For this review, take the finished solid that the model builds, in its own axes (mm). Face numbers are marked on the shaded views. A direction names the side the tool comes from. Give positions to 0.01 mm unless a question says otherwise; leave off trailing zeros. Loops run counter-clockwise (first coordinate to the right, second up) from the corner with the lowest first, then second, coordinate; pieces in that order, holes last. Notation, with made-up numbers: M 67.25,59 L 107.25,59 A16 ccw 107.25,65 Z; hole C -12.75,49 d5. An arc over 180 degrees is marked long. Use CSV: the item, a comma, the result in double quotes. Start each with the question number.
1. Insertion check: P1, Ø2, axis at x = 48.5, y = 26.5, coming from the +Z side; P2, Ø1.5, axis at y = 4.5, z = -7, coming from the -X side (3 decimals); P3, Ø6, axis at y = 18.5, z = -7, coming from the +X side (3 decimals). Each pin has a flat end and moves straight along its axis. Give the tip position at first contact, or say it passes through.
2. Take a section at C-C, the plane y = 7.5. Write out the cut boundary in (x, z) (3 decimals).
3. The part is to be moulded in two halves that separate along Y. For the marked faces 1, 2 and 3, say which applies: pulls with the +Y half, pulls with the -Y half, needs draft (parallel to the pull), parting line crosses it, or undercut.
4. Take a section at D-D, the plane y = -54.5. Write out the cut boundary in (x, z).
5. Take a section at B-B, the plane x = 39. Write out the cut boundary in (y, z), and give its area (3 significant figures).
6. Tool access review of the marked faces 4, 5 and 6: name each direction out of +Z, -Z, +X, -X, +Y, -Y from which nothing blocks a thin tool from reaching the whole face with its end or side.
7. Take a section at A-A, the plane z = -13. Write out the cut boundary in (x, y) (3 decimals), and give its area (3 significant figures).
8. To check wall thickness, follow line 1 (X direction, y = 2, z = -4.25) (3 decimals); line 2 (Y direction, x = -25.5, z = -3.75); line 3 (Z direction, x = 79.5, y = 45). State the ranges of each line that lie inside material, in increasing order. Write a range as [from, to].
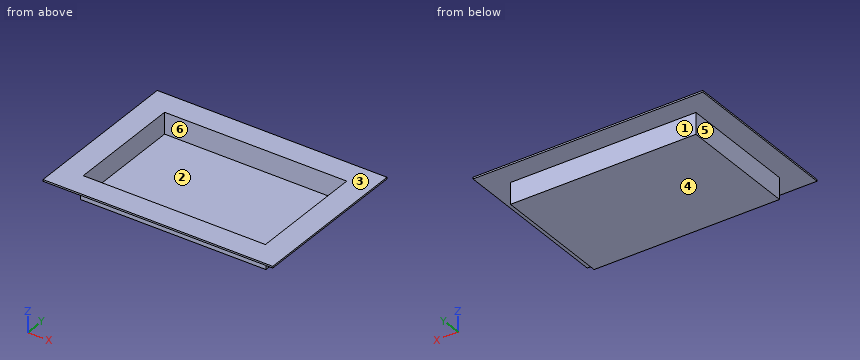
from build123d import *

# Parameters (mm, degrees)
SKETCH1_W           = 143.51
SKETCH1_H           = 92.964
BOSS_EXTRUDE1_DEPTH = 16.51
SKETCH2_W           = 177.8
SKETCH2_H           = 127
BOSS_EXTRUDE2_DEPTH = 1.27
SHELL1_START        = -70.485
SHELL1_OUTLINE_W    = 90.424
SHELL1_OUTLINE_H    = 16.51
SHELL1_DEPTH        = 140.97


# Read off the part's stored shape, not the designer's step: Shell1
with BuildPart() as part:
    # Sketch1 → Boss-Extrude1 (new body)
    with BuildSketch(Plane.XY):
        Rectangle(SKETCH1_W, SKETCH1_H)
    extrude(amount=-BOSS_EXTRUDE1_DEPTH)

    # Sketch2 → Boss-Extrude2 (add)
    with BuildSketch(Plane.XY):
        Rectangle(SKETCH2_W, SKETCH2_H)
    extrude(amount=BOSS_EXTRUDE2_DEPTH)

    # Shell1 outline → Shell1 (cut)
    with BuildSketch(Plane.YZ.offset(SHELL1_START)):
        with Locations((0, -6.985)):
            Rectangle(SHELL1_OUTLINE_W, SHELL1_OUTLINE_H)
    extrude(amount=SHELL1_DEPTH, mode=Mode.SUBTRACT)


solid = part.part
Result set:
1,P1,"z = -15.24"
1,P2,"x = -71.755"
1,P3,"x = 71.755"
2,outline,"M -88.9,0 L -71.755,0 L -71.755,-16.51 L 71.755,-16.51 L 71.755,0 L 88.9,0 L 88.9,1.27 L 70.485,1.27 L 70.485,-15.24 L -70.485,-15.24 L -70.485,1.27 L -88.9,1.27 Z"
3,face 1,"pulls with the +Y half"
3,face 2,"undercut"
3,face 3,"needs draft"
4,outline,"M -88.9,0 L 88.9,0 L 88.9,1.27 L -88.9,1.27 Z"
5,outline,"M -63.5,0 L -46.48,0 L -46.48,-16.51 L 46.48,-16.51 L 46.48,0 L 63.5,0 L 63.5,1.27 L 45.21,1.27 L 45.21,-15.24 L -45.21,-15.24 L -45.21,1.27 L -63.5,1.27 Z"
5,area,"203 mm2"
6,face 4,"-Z, +X, -X, +Y, -Y"
6,face 5,"-Z, -X, +Y, -Y"
6,face 6,"+Z"
7,outline,"M -71.755,-46.482 L 71.755,-46.482 L 71.755,46.482 L -71.755,46.482 Z; hole M -70.485,-45.212 L 70.485,-45.212 L 70.485,45.212 L -70.485,45.212 Z"
7,area,"594 mm2"
8,line 1,"[-71.755, -70.485], [70.485, 71.755]"
8,line 2,"[-46.48, -45.21], [45.21, 46.48]"
8,line 3,"[0, 1.27]"
